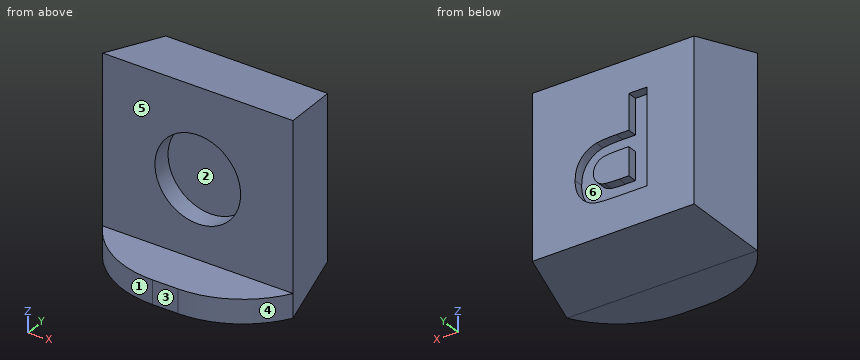
from build123d import *

# Parameters (mm, degrees)
SKETCH1_W               = 8
SKETCH1_H               = 8
BOSS_EXTRUDE1_DEPTH     = 3
CUT_EXTRUDE1_DEPTH      = 12.704699911
CUT_EXTRUDE1_DEPTH_BACK = 12.704699911
CUT_EXTRUDE2_DEPTH      = 11
SKETCH4_R               = 1.8
CUT_EXTRUDE3_DEPTH      = 0.8
SKETCH5_W               = 8
SKETCH5_H               = 1
BOSS_EXTRUDE2_DEPTH     = 2
FILLET1_R               = 4
CUT_EXTRUDE4_DEPTH      = 0.4


with BuildPart() as part:
    # Sketch1 → Boss-Extrude1 (new body)
    with BuildSketch(Plane(origin=(0, 0, 0), x_dir=(1, 0, 0), z_dir=(0, 1, 0))):
        with Locations((4, 4)):
            Rectangle(SKETCH1_W, SKETCH1_H)
    extrude(amount=BOSS_EXTRUDE1_DEPTH)

    # Sketch2 → Cut-Extrude1 (cut, two sides: drawn at the far end of the back side and taken through both)
    with BuildSketch(Plane.XY.offset(-CUT_EXTRUDE1_DEPTH_BACK)):
        Polygon((0, 0), (0.6, 3), (0, 3), align=None)
        Polygon((8, 0), (7.4, 3), (8, 3), align=None)
    extrude(amount=CUT_EXTRUDE1_DEPTH + CUT_EXTRUDE1_DEPTH_BACK, mode=Mode.SUBTRACT)

    # Sketch3 → Cut-Extrude2 (cut)
    with BuildSketch(Plane(origin=(0, 0, 0), x_dir=(0, 0, -1), z_dir=(1, 0, 0))):
        Polygon((0, 0), (0.6, 3), (0, 3), align=None)
        Polygon((8, 3), (7.4, 3), (8, 0), align=None)
    extrude(amount=CUT_EXTRUDE2_DEPTH, mode=Mode.SUBTRACT)

    # Sketch4 → Cut-Extrude3 (cut)
    with BuildSketch(Plane.XZ):
        with Locations(Location((4, -3.75, 0), (0, 0, 270))):
            Circle(SKETCH4_R)
    extrude(amount=-CUT_EXTRUDE3_DEPTH, mode=Mode.SUBTRACT)

    # Sketch5 → Boss-Extrude2 (add)
    with BuildSketch(Plane.XZ):
        with Locations((4, -7.5)):
            Rectangle(SKETCH5_W, SKETCH5_H)
    extrude(amount=BOSS_EXTRUDE2_DEPTH)

    # Fillet1
    # the kernel refuses this fillet: 4 mm, written as the material it takes off along each edge
    with BuildSketch(Plane(origin=(8, -2, -16.660254038), x_dir=(0, 1, 0), z_dir=(0, 0, 1)), Plane(origin=(0, -2, 1.660254038), x_dir=(0, 1, 0), z_dir=(0, 0, -1))) as fillet1_piece_1:
        with BuildLine():
            CenterArc((4, 3.464101615), FILLET1_R, 180, 60)
            Line((0, 3.464101615), (-0.08, 3.464101615))
            Line((-0.08, 3.464101615), (-0.08, 0))
            Line((-0.08, 0), (0, -0.08))
            ThreePointArc((0, -0.08), (1, -0.08), (1.96, -0.069282032))
            Line((1.96, -0.069282032), (2, 0))
        make_face()
    extrude(amount=18.320508076, mode=Mode.SUBTRACT)

    # Sketch6 → Cut-Extrude4 (cut)
    with BuildSketch(Plane(origin=(0, 3, 0), x_dir=(1, 0, 0), z_dir=(0, 1, 0))):
        with BuildLine():
            Line((2.575068598, 1.987434605), (2.575068598, 5.987434605))
            Line((2.575068598, 5.987434605), (3.854716034, 5.987434605))
            add(Edge.make_bspline(
                [(3.854716034, 5.987434605), (3.91267733, 5.987371309), (4.0235352, 5.987250247), (4.181667245, 5.983886636), (4.324041461, 5.979125075), (4.450446542, 5.973194752), (4.561327274, 5.964345571), (4.656186257, 5.954098352), (4.735620814, 5.943075064), (4.782397472, 5.931667436), (4.803433983, 5.926537169)],
                knots=[0, 0, 0, 0, 1.460485487, 2.793352117, 3.985295279, 5.050041172, 5.981765236, 6.787433016, 7.454681457, 8, 8, 8, 8], degree=3))
            add(Edge.make_bspline(
                [(4.803433983, 5.926537169), (4.831407427, 5.918560862), (4.886928159, 5.902729762), (4.966472056, 5.868980371), (5.043139776, 5.829866627), (5.115968073, 5.783250114), (5.185204512, 5.72995844), (5.251054895, 5.670426205), (5.313870394, 5.604384669), (5.372782037, 5.531964292), (5.426738172, 5.453530256), (5.473369829, 5.368966598), (5.512437408, 5.278640875), (5.545722335, 5.183231873), (5.570280113, 5.081716653), (5.587466094, 4.974800554), (5.59942968, 4.862436815), (5.600276739, 4.785544235), (5.600709624, 4.746248708)],
                knots=[0, 0, 0, 0, 0.907145743, 1.80047177, 2.69161667, 3.591261238, 4.495029544, 5.415863088, 6.359363025, 7.337192411, 8.326890979, 9.326929023, 10.346104993, 11.395420813, 12.477187422, 13.601053412, 14.774031606, 16, 16, 16, 16], degree=3))
            add(Edge.make_bspline(
                [(5.600709624, 4.746248708), (5.599475039, 4.686573982), (5.597098394, 4.571696857), (5.570507962, 4.407006575), (5.529951011, 4.256572619), (5.470674098, 4.121843981), (5.398403226, 4.002291963), (5.318795373, 3.894516382), (5.227894903, 3.801765706), (5.129684965, 3.722543108), (5.025895009, 3.65771062), (4.921917172, 3.602441845), (4.816348426, 3.559949444), (4.744371889, 3.541435164), (4.708882701, 3.5323064)],
                knots=[0, 0, 0, 0, 1.312386234, 2.526415563, 3.661883817, 4.733421185, 5.753802465, 6.732107337, 7.675884281, 8.604170108, 9.50284679, 10.365392406, 11.194030444, 12, 12, 12, 12], degree=3))
            add(Edge.make_bspline(
                [(4.708882701, 3.5323064), (4.683552258, 3.527487955), (4.630158709, 3.517331247), (4.545479732, 3.507206857), (4.452921022, 3.496000262), (4.352101878, 3.488690691), (4.243144264, 3.481845584), (4.126090489, 3.478613784), (4.001107836, 3.47472012), (3.91508314, 3.474650156), (3.870741675, 3.474614092)],
                knots=[0, 0, 0, 0, 0.735353946, 1.55003838, 2.431865514, 3.394945452, 4.432993119, 5.54609699, 6.735134699, 8, 8, 8, 8], degree=3))
            Line((3.870741675, 3.474614092), (3.344299367, 3.474614092))
            Line((3.344299367, 3.474614092), (3.344299367, 1.987434605))
            Line((3.344299367, 1.987434605), (2.575068598, 1.987434605))
        make_face()
        with BuildLine():
            Line((3.344299367, 5.320767939), (3.344299367, 4.141280759))
            Line((3.344299367, 4.141280759), (3.805837829, 4.141280759))
            add(Edge.make_bspline(
                [(3.805837829, 4.141280759), (3.845638333, 4.141332297), (3.921781705, 4.141430897), (4.031030553, 4.144970031), (4.129922714, 4.149290201), (4.218664819, 4.156440966), (4.296721198, 4.165865503), (4.364614575, 4.177138437), (4.422424078, 4.189235472), (4.484937186, 4.209282199), (4.551776196, 4.241715975), (4.623152404, 4.288331456), (4.685856319, 4.344065763), (4.738034287, 4.409523776), (4.779712931, 4.482251421), (4.809554871, 4.56150336), (4.828823783, 4.645966113), (4.830583823, 4.704475652), (4.831478855, 4.734229477)],
                knots=[0, 0, 0, 0, 1.411705958, 2.700771114, 3.876961699, 4.922619712, 5.858038221, 6.66485904, 7.363650596, 7.950905807, 8.989198271, 9.987739806, 10.967313358, 11.951275539, 12.944273208, 13.927870418, 14.946261014, 16, 16, 16, 16], degree=3))
            add(Edge.make_bspline(
                [(4.831478855, 4.734229477), (4.830219195, 4.770469172), (4.827776882, 4.840733161), (4.800844983, 4.940800809), (4.759292142, 5.031613413), (4.699883375, 5.110345382), (4.628118983, 5.176552494), (4.547458802, 5.231639165), (4.456180297, 5.270189236), (4.391579581, 5.285125966), (4.358722444, 5.292723067)],
                knots=[0, 0, 0, 0, 1.085904563, 2.105425768, 3.088705091, 4.068969419, 5.045188284, 6.010769642, 6.988240112, 8, 8, 8, 8], degree=3))
            add(Edge.make_bspline(
                [(4.358722444, 5.292723067), (4.344583268, 5.294984513), (4.31319868, 5.300004222), (4.261031108, 5.305242912), (4.199316862, 5.310007496), (4.127981551, 5.313919362), (4.047307931, 5.316977535), (3.957029905, 5.319657249), (3.857385235, 5.319872528), (3.787674783, 5.320461199), (3.751350649, 5.320767939)],
                knots=[0, 0, 0, 0, 0.564603001, 1.253243608, 2.066786758, 3.005752288, 4.070476343, 5.250658742, 6.567396469, 8, 8, 8, 8], degree=3))
            Line((3.751350649, 5.320767939), (3.344299367, 5.320767939))
        make_face(mode=Mode.SUBTRACT)
    extrude(amount=-CUT_EXTRUDE4_DEPTH, mode=Mode.SUBTRACT)


solid = part.part
Source: CAD feature listing. Evaluate the final solid. Frame: model axes, mm. Face numbers are marked on the shaded views. A direction names the side the tool comes from. Coordinates: 2 decimals unless noted, no trailing zeros. Loops run counter-clockwise (first coordinate to the right, second up) from the corner with the lowest first, then second, coordinate; pieces in that order, holes last. Notation, with made-up numbers: (33.5, -23.75) -> (47.5, -23.75) arc R4 cw to (47.5, -18.75) -> close; hole circle Ø7 at (46.5, 83). An arc over 180 degrees is marked (long way). Answer in a Markdown table with one row per item. Add a question column.
Q1. Reachability of the marked faces 4, 5 and 6 from +Z, -Z, +X, -X, +Y, -Y: full face, straight path, thin tool, end or side. Return the list, or none.
Q2. Section B-B on z = -6.5. Return the cut outline in (x, y).
Q3. Section D-D on y = 1.5. Return the cut outline in (x, z), and give its area (3 significant figures).
Q4. Section C-C on x = 6.25. Return the cut outline in (y, z).
Q5. Section A-A on y = 0.55. Return the cut outline in (x, z), and give its area (3 significant figures).
Q6. Pull-direction query (X, two-part tool) for the marked faces 1, 2 and 3; classes: pulls with the +X half, pulls with the -X half, needs draft (parallel to the pull), parting line crosses it, or undercut.
Q7. Contact query for flat-ended pins moving along their axis: pin 1 Ø2 at (x, z) = (2, -3.5) entering from -Y; pin 2 Ø3 at (x, z) = (4, -3.75) entering from -Y; pin 3 Ø0.6 at (x, y) = (3, -1) entering from +Z. Output: stop coordinate, or through.
Q8. Ray query, line 1 along Y through (x, z) = (6.5, -6.25); line 2 along X through (y, z) = (0.35, -3.75); line 3 along X through (y, z) = (0.5, -2.25). Return the intervals inside material, ascending.
Computed values:
| question | item | result |
|---|---|---|
| 1 | face 4 | +Z, -Z, +X, -Y |
| 1 | face 5 | +Z, +X, -X, -Y |
| 1 | face 6 | +Y |
| 2 | outline | (0, 0) -> (8, 0) -> (7.4, 3) -> (0.6, 3) -> close |
| 3 | outline | (0.3, -7.7) -> (7.7, -7.7) -> (7.7, -0.3) -> (0.3, -0.3) -> close |
| 3 | area | 54.8 mm^2 |
| 4 | outline | (-1.61, -8) -> (0, -8) -> (3, -7.4) -> (3, -0.6) -> (0, 0) -> (0, -7) -> (-1.61, -7) -> close |
| 5 | outline | (0.11, -7.89) -> (7.89, -7.89) -> (7.89, -0.11) -> (0.11, -0.11) -> close; hole circle Ø3.6 at (4, -3.75) |
| 5 | area | 50.3 mm^2 |
| 6 | face 1 | pulls with the -X half |
| 6 | face 2 | undercut |
| 6 | face 3 | needs draft |
| 7 | pin 1 | stops at y = 0 |
| 7 | pin 2 | stops at y = 0.8 |
| 7 | pin 3 | stops at z = -7 |
| 8 | line 1 | y = 0 to 3 |
| 8 | line 2 | x = 0.07 to 2.2, 5.8 to 7.93 |
| 8 | line 3 | x = 0.1 to 3.01, 4.99 to 7.9 |
